```python
from build123d import *

# Parameters (mm, degrees)
SKETCH3_W                                    = 25.4
SKETCH3_H                                    = 6
BOSS_EXTRUDE1_DEPTH                          = 182
CSK_FOR_1_4_FLAT_HEAD_SOCKET_CAP_SCR_2_COUNT = 2
CSK_FOR_1_4_FLAT_HEAD_SOCKET_CAP_SCR_2_PITCH = 338.6
CSK_FOR_1_4_FLAT_HEAD_SOCKET_CAP_SCR_3_COUNT = 2
CSK_FOR_1_4_FLAT_HEAD_SOCKET_CAP_SCR_3_PITCH = 50.8
CSK_FOR_1_4_FLAT_HEAD_SOCKET_CAP_SCR_4_COUNT = 2
CSK_FOR_1_4_FLAT_HEAD_SOCKET_CAP_SCR_4_PITCH = 287.8


with BuildPart() as part:
    # Sketch3 → Boss-Extrude1 (new body, symmetric)
    with BuildSketch(Plane.XY):
        Rectangle(SKETCH3_W, SKETCH3_H)
    extrude(amount=BOSS_EXTRUDE1_DEPTH, both=True)

    # Sketch8 → CSK for 1/4 Flat Head Socket Cap Screw1 (revolve, cut)
    with BuildSketch(Plane(origin=(0, 3, -169.3), x_dir=(0, 0, 1), z_dir=(1, 0, 0))):
        Polygon((0, 0), (0, 6), (3.3782, 6), (3.3782, 4.371566521), (7.1783448, 0), align=None)
    csk_for_1_4_flat_head_socket_cap_screw1 = revolve(axis=Axis((0, 9.35, -169.3), (0, -1, 0)), mode=Mode.SUBTRACT)

    # CSK for 1_4 Flat Head Socket Cap Scr 2: CSK for 1/4 Flat Head Socket Cap Screw1 ×2
    with Locations(*[(0, 0, i * CSK_FOR_1_4_FLAT_HEAD_SOCKET_CAP_SCR_2_PITCH) for i in range(1, CSK_FOR_1_4_FLAT_HEAD_SOCKET_CAP_SCR_2_COUNT)]):
        add(csk_for_1_4_flat_head_socket_cap_screw1, mode=Mode.SUBTRACT)

    # CSK for 1_4 Flat Head Socket Cap Scr 3: CSK for 1/4 Flat Head Socket Cap Screw1 ×2
    with Locations(*[(0, 0, i * CSK_FOR_1_4_FLAT_HEAD_SOCKET_CAP_SCR_3_PITCH) for i in range(1, CSK_FOR_1_4_FLAT_HEAD_SOCKET_CAP_SCR_3_COUNT)]):
        add(csk_for_1_4_flat_head_socket_cap_screw1, mode=Mode.SUBTRACT)

    # CSK for 1_4 Flat Head Socket Cap Scr 4: CSK for 1/4 Flat Head Socket Cap Screw1 ×2
    with Locations(*[(0, 0, i * CSK_FOR_1_4_FLAT_HEAD_SOCKET_CAP_SCR_4_PITCH) for i in range(1, CSK_FOR_1_4_FLAT_HEAD_SOCKET_CAP_SCR_4_COUNT)]):
        add(csk_for_1_4_flat_head_socket_cap_screw1, mode=Mode.SUBTRACT)


solid = part.part
```
Geometry check sheet. Reference: the model listing, model coordinates, mm. Give positions to 0.01 mm unless a question says otherwise; leave off trailing zeros. Order: outer loops, then holes, each group sorted by start corner. A loop starts at its lowest first (then second) coordinate and runs counter-clockwise, first axis right, second up.
1. Section check A-A, the plane x = 0. Enter the section's corners in (y, z), and give its area (3 significant figures).
2. Gauge pin test, flat ends, axial feed: pin 1 Ø4 at (x, z) = (0, 118.5) entering from -Y; pin 2 Ø11 at (x, z) = (0, -169.3) entering from +Y. Record the tip position at first contact, or that the pin passes through.
3. Thickness scan on L1, parallel to Z at x = 0, y = -2.05; L2, parallel to X at y = -2.35, z = 169.3; L3, parallel to Z at x = 4, y = 1.2. Record the ranges inside material, lowest first.
4. Release check for a two-part mould opening along X. For faces 1 (the face through (-12.7, 0, 3)), 2 (the face through (12.7, 0, 3)), 3 (the face through (2.2, -1.1, 115.63)), 4 (the face through (0, 3, 3)) record: pulls with the +X half, pulls with the -X half, needs draft (parallel to the pull), parting line crosses it, or undercut.
5. Section check B-B, the plane z = -118.5. Enter the section's corners in (x, y).
6. Section check C-C, the plane y = 0.8. Enter the section's corners in (x, z), and give its area (3 significant figures).
Values follow:
1. outline: (-3, -182) - (3, -182) - (3, -176.48) - (-1.37, -172.68) - (-3, -172.68) - close; (-3, -165.92) - (-1.37, -165.92) - (3, -162.12) - (3, -125.68) - (-1.37, -121.88) - (-3, -121.88) - close; (-3, -115.12) - (-1.37, -115.12) - (3, -111.32) - (3, 111.32) - (-1.37, 115.12) - (-3, 115.12) - close; (-3, 121.88) - (-1.37, 121.88) - (3, 125.68) - (3, 162.12) - (-1.37, 165.92) - (-3, 165.92) - close; (-3, 172.68) - (-1.37, 172.68) - (3, 176.48) - (3, 182) - (-3, 182) - close
1. area: 1,960 mm2
2. pin 1: passes through
2. pin 2: stops at y = 1.07
3. L1: z = -182 to -172.68, -165.92 to -121.88, -115.12 to 115.12, 121.88 to 165.92, 172.68 to 182
3. L2: x = -12.7 to -3.38, 3.38 to 12.7
3. L3: z = -182 to -173.24, -165.36 to -122.44, -114.56 to 114.56, 122.44 to 165.36, 173.24 to 182
4. face 1: pulls with the -X half
4. face 2: pulls with the +X half
4. face 3: undercut
4. face 4: needs draft
5. outline: (-12.7, -3) - (-3.38, -3) - (-3.38, -1.37) - (-7.18, 3) - (-12.7, 3) - close; (3.38, -3) - (12.7, -3) - (12.7, 3) - (7.18, 3) - (3.38, -1.37) - close
6. outline: (-12.7, -182) - (12.7, -182) - (12.7, 182) - (-12.7, 182) - close; hole circle Ø10.53 at (0, -169.3); hole circle Ø10.53 at (0, -118.5); hole circle Ø10.53 at (0, 118.5); hole circle Ø10.53 at (0, 169.3)
6. area: 8,900 mm2
